Could you check a few things on this model? Use its own coordinates, in mm. Coordinates: 2 decimals unless noted, no trailing zeros. Order: outer loops, then holes, each group sorted by start corner. A loop starts at its lowest first (then second) coordinate and runs counter-clockwise, first axis right, second up. Notation, with made-up numbers: (80.25, 52) - (129.25, 52) arc R20 ccw to (129.25, 79) - close; hole circle Ø11 at (63, -9.75). An arc over 180 degrees is marked (long way). One line per item, written item: value.
from build123d import *

# Parameters (mm, degrees)
RESSALTO_EXTRUS_O2_DEPTH = 6
RESSALTO_EXTRUS_O3_DEPTH = 6
CORTE_EXTRUS_O2_DEPTH    = 10
ESBO_O7_W                = 235.908254568
ESBO_O7_H                = 6
RESSALTO_EXTRUS_O4_DEPTH = 253
ESBO_O8_W                = 6.266008042
ESBO_O8_H                = 6
CORTE_EXTRUS_O3_DEPTH    = 6
ESBO_O9_R                = 3
CORTE_EXTRUS_O4_DEPTH    = 342.610457354
ESBO_O10_R               = 3
CORTE_EXTRUS_O5_DEPTH    = 553.891223092


with BuildPart() as part:
    # Esboço1 → Ressalto-extrusão2 (new body)
    with BuildSketch(Plane.XY):
        with BuildLine():
            Line((-199.999999999, 0), (199.999999999, 0))
            ThreePointArc((199.999999999, 0), (202.565835097, -15.811388301), (209.999999999, -30))
            Line((209.999999999, -30), (289.999999999, -30))
            ThreePointArc((289.999999999, -30), (299.999014124, 0.31398499), (289.62007067, 30.5))
            ThreePointArc((289.62007067, 30.5), (297.818976076, 75.60635228), (265.815415017, 108.432822474))
            Line((265.815415017, 108.432822474), (246.403986634, 35.988385502))
            ThreePointArc((246.403986634, 35.988385502), (242.72975202, 33.867065158), (240.608431676, 37.541299773))
            Line((240.608431676, 37.541299773), (260.019860059, 109.985736744))
            ThreePointArc((260.019860059, 109.985736744), (218.38507475, 99.736242739), (199.999999999, 61))
            Line((199.999999999, 61), (140, 61))
            Line((140, 61), (150.784643454, 58.387579086))
            Line((150.784643454, 58.387579086), (139.047219324, 52.742194858))
            Line((139.047219324, 52.742194858), (160.085396074, 40.245061921))
            Line((160.085396074, 40.245061921), (137.597498913, 43.437533109))
            Line((137.597498913, 43.437533109), (153.154101004, 34.194272541))
            Line((153.154101004, 34.194272541), (138.26257587, 30.30469508))
            Line((138.26257587, 30.30469508), (144.152507453, 26))
            Line((144.152507453, 26), (149.999999999, 26))
            ThreePointArc((149.999999999, 26), (152.999999999, 23), (149.999999999, 20))
            Line((149.999999999, 20), (-149.999999999, 20))
            ThreePointArc((-149.999999999, 20), (-152.999999999, 23), (-149.999999999, 26))
            Line((-149.999999999, 26), (-144.152507453, 26))
            Line((-144.152507453, 26), (-138.26257587, 30.30469508))
            Line((-138.26257587, 30.30469508), (-153.154101004, 34.194272541))
            Line((-153.154101004, 34.194272541), (-137.597498913, 43.437533109))
            Line((-137.597498913, 43.437533109), (-160.085396074, 40.245061921))
            Line((-160.085396074, 40.245061921), (-139.047219324, 52.742194858))
            Line((-139.047219324, 52.742194858), (-150.784643454, 58.387579086))
            Line((-150.784643454, 58.387579086), (-140, 61))
            Line((-140, 61), (-199.999999999, 61))
            ThreePointArc((-199.999999999, 61), (-218.38507475, 99.736242739), (-260.019860059, 109.985736744))
            Line((-260.019860059, 109.985736744), (-240.608431676, 37.541299773))
            ThreePointArc((-240.608431676, 37.541299773), (-242.72975202, 33.867065158), (-246.403986634, 35.988385502))
            Line((-246.403986634, 35.988385502), (-265.815415017, 108.432822474))
            ThreePointArc((-265.815415017, 108.432822474), (-297.818976076, 75.60635228), (-289.62007067, 30.5))
            ThreePointArc((-289.62007067, 30.5), (-299.999014124, 0.31398499), (-289.999999999, -30))
            Line((-289.999999999, -30), (-209.999999999, -30))
            ThreePointArc((-209.999999999, -30), (-202.565835097, -15.811388301), (-199.999999999, 0))
        make_face()
    extrude(amount=RESSALTO_EXTRUS_O2_DEPTH)

    # Esboço5 → Corte-extrusão2 (cut)
    with BuildSketch(Plane.XY.offset(6)):
        Polygon((-341.805819903, 0), (-379.563439543, 0), (-379.563439543, 200.23140607), (0, 200.23140607), (0, 0), (-124.202696186, 0), (-124.202696186, -126.67009029), (-341.805819903, -126.67009029), align=None)
    extrude(amount=-CORTE_EXTRUS_O2_DEPTH, mode=Mode.SUBTRACT)


with BuildPart() as body_2:
    # Esboço4 → Ressalto-extrusão3 (new body)
    with BuildSketch(Plane(origin=(215.105397993, -57.63731768, 0), x_dir=(0, 0, -1), z_dir=(0.9659258262890679, -0.25881904510252246, 0))):
        with BuildLine():
            Line((246.999999999, 62.536155533), (246.999999999, 123.536155533))
            Line((246.999999999, 123.536155533), (47, 123.536155533))
            ThreePointArc((47, 123.536155533), (32.355339059, 158.891494592), (-3, 173.536155533))
            ThreePointArc((-3, 173.536155533), (-47.860896112, 145.615557699), (-42.620070671, 93.036155533))
            ThreePointArc((-42.620070671, 93.036155533), (-52.987511897, 61.418723482), (-41.217566642, 30.296155533))
            Line((-41.217566642, 30.296155533), (35.217566642, 30.296155533))
            ThreePointArc((35.217566642, 30.296155533), (43.96210351, 45.373380875), (47, 62.536155533))
            Line((47, 62.536155533), (246.999999999, 62.536155533))
        make_face()
    extrude(amount=RESSALTO_EXTRUS_O3_DEPTH)


with BuildPart() as body_3:
    # Esboço7 → Ressalto-extrusão4 (new body)
    with BuildSketch(Plane.XY.offset(6)):
        with Locations((117.954127284, 23)):
            Rectangle(ESBO_O7_W, ESBO_O7_H)
    extrude(amount=-RESSALTO_EXTRUS_O4_DEPTH)

    # Combinar1: cut part, body 2
    add(part.part, mode=Mode.SUBTRACT)
    add(body_2.part, mode=Mode.SUBTRACT)

    # Esboço8 → Corte-extrusão3 (cut)
    with BuildSketch(Plane.XY.offset(6)):
        with Locations((153.13300402, 23)):
            Rectangle(ESBO_O8_W, ESBO_O8_H)
    extrude(amount=-CORTE_EXTRUS_O3_DEPTH, mode=Mode.SUBTRACT)

    # Esboço9 → Corte-extrusão4 (cut, through all)
    with BuildSketch(Plane(origin=(0, 26, 0), x_dir=(1, 0, 0), z_dir=(0, 1, 0))):
        with Locations(Location((225.908254568, 38.284271247, 0), (0, 0, 270))):
            Circle(ESBO_O9_R)
        with Locations(Location((197.623983321, 10, 0), (0, 0, 270))):
            Circle(ESBO_O9_R)
        with Locations(Location((71.161943972, 70.690502615, 0), (0, 0, 270))):
            Circle(ESBO_O9_R)
        with Locations(Location((132.122360106, 70.690502615, 0), (0, 0, 270))):
            Circle(ESBO_O9_R)
        with Locations(Location((71.161943972, 182.100918308, 0), (0, 0, 270))):
            Circle(ESBO_O9_R)
        with Locations(Location((132.122360106, 182.100918308, 0), (0, 0, 270))):
            Circle(ESBO_O9_R)
    extrude(amount=-CORTE_EXTRUS_O4_DEPTH, mode=Mode.SUBTRACT)

    # Espelhar1: body 3 across plane


with BuildPart() as body_3_1:
    add(body_3.part)
    add(body_3.part.mirror(Plane(origin=(0, 26, -246.999999999), x_dir=(0, 0, 1), z_dir=(-1, 0, 0))))

    # Espelhar3: body 3 across plane


with BuildPart() as body_3_2:
    add(body_3_1.part)
    add(body_3_1.part.mirror(Plane.XY.offset(-246.999999999)))

    # Esboço10 → Corte-extrusão5 (cut, through all)
    with BuildSketch(Plane(origin=(0, 20, 0), x_dir=(-1, 0, 0), z_dir=(0, -1, 0))):
        with Locations((149.999999999, 0)):
            Circle(ESBO_O10_R)
        with Locations((-149.999999999, 0)):
            Circle(ESBO_O10_R)
        with Locations((-149.999999999, 493.999999998)):
            Circle(ESBO_O10_R)
        with Locations((149.999999999, 493.999999998)):
            Circle(ESBO_O10_R)
    extrude(amount=-CORTE_EXTRUS_O5_DEPTH, mode=Mode.SUBTRACT)


solid = body_3_2.part
Item 1: If I drill on probe 1 along Z at (x, y) = (-129.5, 20.35); probe 2 along X at (y, z) = (22.6, -314.5); probe 3 along Z at (x, y) = (-170, 25.25), over which ranges is the centre line in solid material (lowest first)?
Conclusion:
probe 1: -500 to -424.77, -421.85 to -313.36, -310.44 to -183.56, -180.64 to -72.15, -69.23 to 6
probe 2: -235.91 to -133.62, -130.63 to -72.66, -69.67 to 69.67, 72.66 to 130.63, 133.62 to 235.91
probe 3: -494 to 0
Item 2: I'm going to push flat-ended pins straight in: pin 1 Ø1.8 at (x, y) = (-193, 22.5) entering from +Z; pin 2 Ø5.5 at (x, z) = (132.12, -311.9) entering from -Y; pin 3 Ø0.9 at (y, z) = (23, -499) entering from -X; pin 4 Ø3 at (x, y) = (203, 23.5) entering from -Z. Where does each tip first touch, or does it pass through?
Conclusion:
pin 1: z = 0
pin 2: through
pin 3: x = -150
pin 4: z = -494
Item 3: I want a section at A-A on x = 165.5. Please give me the cut outline in (y, z), then the cut area to 3 significant figures.
Conclusion:
outline: (20, -494) - (26, -494) - (26, 0) - (20, 0) - close
area: 2,960 mm²
